For this review, take the finished solid that the model builds, in its own axes (mm). A direction names the side the tool comes from. Round coordinates to 2 decimals unless told otherwise and drop trailing zeros. Loops run counter-clockwise (first coordinate to the right, second up) from the corner with the lowest first, then second, coordinate; pieces in that order, holes last.
1) Take a section at B-B (y = 3). State the section outline as (x, z) points (1 decimal).
2) Take a section at A-A (y = -0.65). State the section outline as (x, z) points.
3) Insertion check: pin 1 (5.5 mm diameter, centred on x = 0, z = 0, fed in from +Y); pin 2 (3 mm diameter, centred on x = 3, y = -1.5, fed in from -Z); pin 3 (3 mm diameter, centred on x = -2, y = 2, fed in from -Z). Each pin has a flat end and moves straight along its axis. Give the tip position at first contact, or say it passes through.
4) Mouldability with a two-part tool opening along X and no side actions: class faces 1 (the conical face through (-4.27, 1.81, 2.48)), 2 (the cylindrical face through (1.926, 0.951, 0.607)), 3 (the flat face through (2.41, 0.03, -4.11)), 4 (the conical face through (0.01, 1.81, 4.94)) as pulls with the +X half, pulls with the -X half, needs draft (parallel to the pull), parting line crosses it, or undercut.
5) Tool access review of faces 5 (the conical face through (-4.27, -1.81, 2.48)), 6 (the cylindrical face through (-3.78, 2.84, 2.9)): name each direction out of +Z, -Z, +X, -X, +Y, -Y from which nothing blocks a thin tool from reaching the whole face with its end or side.
6) Wall thickness on L1, parallel to Z at x = -0.25, y = 2.9; L2, parallel to Z at x = 0.5, y = 1.45; L3, parallel to Z at x = -4.25, y = 3.75: over which ranges is each line inside the solid? List them lowest first.
```python
from build123d import *

# Parameters (mm, degrees)
EXTRUDE1_DEPTH              = 1.98501
SKETCH2_OUTSIDE_W           = 22.481
SKETCH2_OUTSIDE_H           = 23.954
SKETCH2_OUTSIDE_R           = 4.7625
EXTRUDE3_DEPTH              = 3.97002
EXTRUDE3_TAPER              = 45
SKETCH3_R                   = 4.7625
EXTRUDE4_DEPTH              = 1.984375
F_21_0_159_DIAMETER_HOLE1_D = 4.0386
CHAMFER1_SIZE               = 0.254


with BuildPart() as part:
    # Sketch1 → Extrude1 (new body, symmetric)
    with BuildSketch(Plane(origin=(0, 0, 0), x_dir=(1, 0, 0), z_dir=(0, 1, 0))):
        Polygon((0, 5.499261314), (-4.7625, 2.749630657), (-4.7625, -2.749630657), (0, -5.499261314), (4.7625, -2.749630657), (4.7625, 2.749630657), align=None)
    extrude(amount=EXTRUDE1_DEPTH, both=True)

    # Sketch2 outside → Extrude3 (cut)
    with BuildSketch(Plane(origin=(0, 1.98501, 0), x_dir=(1, 0, 0), z_dir=(0, 1, 0))):
        with Locations((-0.0005, 0)):
            Rectangle(SKETCH2_OUTSIDE_W, SKETCH2_OUTSIDE_H)
        Circle(SKETCH2_OUTSIDE_R, mode=Mode.SUBTRACT)
    extrude3 = extrude(amount=-EXTRUDE3_DEPTH, taper=EXTRUDE3_TAPER, mode=Mode.SUBTRACT)

    # Mirror1: Extrude3 across plane
    add(extrude3.mirror(Plane.ZX), mode=Mode.SUBTRACT)

    # Sketch3 → Extrude4 (add)
    with BuildSketch(Plane(origin=(0, 1.98501, 0), x_dir=(1, 0, 0), z_dir=(0, 1, 0))):
        Circle(SKETCH3_R)
    extrude(amount=EXTRUDE4_DEPTH)

    # #21 (0.159) Diameter Hole1 (through all)
    with Locations(Plane(origin=(0, 3.969385, 0), x_dir=(-1, 0, 0), z_dir=(0, 1, 0))):
        with Locations((0, 0)):
            Hole(F_21_0_159_DIAMETER_HOLE1_D / 2)

    # Chamfer1
    chamfer1_edges = [part.edges().sort_by_distance(p)[0] for p in [
        (-4.7625, 3.969385, 0),
    ]]
    chamfer(chamfer1_edges, length=CHAMFER1_SIZE)


solid = part.part
```
Response:
1. outline: circle Ø9.5 at (0, 0); hole circle Ø4 at (0, 0)
2. outline: (-4.76, -2.75) - (0, -5.5) - (4.76, -2.75) - (4.76, 2.75) - (0, 5.5) - (-4.76, 2.75) - close; hole circle Ø4.04 at (0, 0)
3. pin 1: stops at y = 3.97
3. pin 2: stops at z = -4.63
3. pin 3: stops at z = -5.17
4. face 1: pulls with the -X half
4. face 2: undercut
4. face 3: pulls with the +X half
4. face 4: parting line crosses it
5. face 5: +Z, -X, -Y
5. face 6: +Y
6. L1: z = -4.76 to -2, 2 to 4.76
6. L2: z = -5.21 to -1.96, 1.96 to 5.21
6. L3: z = -2.07 to 2.07
